Autodesk Inventor part; units mm, degrees
ref_plane "YZ Plane" through (0, 0, 0) normal (1, 0, 0) x (0, 1, 0)
ref_plane "XZ Plane" through (0, 0, 0) normal (0, 1, 0) x (-1, 0, 0)
ref_plane "XY Plane" through (0, 0, 0) normal (0, 0, 1) x (1, 0, 0)
sketch "スケッチ1" plane through (0, 0, 0) normal (0, 0, 1) x (1, 0, 0)
  circle A0 centre (0, 0) radius 17.9
  dimension "d0" = 35.8
extrude "押し出し1" add sketch "スケッチ1" against normal blind 3.3
fillet "フィレット1" radius 3 1 edges at (-17.9, 0, 0)
sketch "スケッチ2" plane through (0, 0, -3.3) normal (0, 0, -1) x (-1, 0, 0)
  circle A0 centre (0, 0) radius 19.25
  dimension "d4" = 38.5
extrude "押し出し2" add sketch "スケッチ2" along normal blind 38
sketch "スケッチ3" plane through (0, 0, -41.3) normal (0, 0, -1) x (-1, 0, 0)
  circle A0 centre (0, 0) radius 17.9
  dimension "d7" = 35.8
extrude "押し出し3" add sketch "スケッチ3" along normal blind 15.7
sketch "スケッチ4" plane through (0, 0, -57) normal (0, 0, -1) x (-1, 0, 0)
  circle A0 centre (0, 0) radius 1.585
  dimension "d10" = 3.17
extrude "押し出し4" add sketch "スケッチ4" along normal blind 10.7
sketch "スケッチ5" plane through (0, 0, 0) normal (0, 0, 1) x (1, 0, 0)
  circle A0 centre (0, 0) radius 1.585
  circle A1 centre (0, 0) radius 16
  dimension "d13" = 32
extrude "押し出し5" add sketch "スケッチ5" along normal blind 34.9 contours A0 | A1
chamfer "面取り1" distance 1 angle 45 1 edges at (-16, 0, 34.9)
sketch "スケッチ6" plane through (0, 0, 34.9) normal (0, 0, 1) x (1, 0, 0)
  circle A0 centre (0, 0) radius 10
  dimension "d19" = 20
extrude "押し出し6" add sketch "スケッチ6" along normal blind 3
sketch "スケッチ7" plane through (0, 0, 37.9) normal (0, 0, 1) x (1, 0, 0)
  circle A0 centre (0, 0) radius 1.585
  circle A1 centre (0, 0) radius 3
  dimension "d22" = 6
extrude "押し出し7" add sketch "スケッチ7" along normal blind 16.3 contours A0 | A1
sketch "スケッチ8" plane through (0, 0, 54.2) normal (0, 0, 1) x (1, 0, 0)
  circle A0 centre (0, 0) radius 3
  line L0 (-1.6583, 2.5) -> (1.6583, 2.5)
  arc A1 (1.6583, 2.5) -> (-1.6583, 2.5) centre (0, 0) ccw
  dimension "d25" = 2.5
extrude "押し出し8" cut sketch "スケッチ8" against normal blind 12 contours L0 A0 picked at (-0.1169, 2.6598)
sketch "スケッチ9" plane through (0, 0, 34.9) normal (0, 0, 1) x (1, 0, 0)
  circle A0 centre (0, 13) radius 1.25
  circle A1 centre (-13, 0) radius 1.25
  circle A2 centre (0, -13) radius 1.25
  circle A3 centre (13, 0) radius 1.25
  circle A4 centre (0, 0) radius 13 construction
  dimension "d28" = 2.5
  dimension "d29" = 2.5
  dimension "d30" = 2.5
  dimension "d31" = 2.5
  dimension "d32" = 26
extrude "押し出し9" cut sketch "スケッチ9" against normal blind 12
properties part number "RS-555-71"
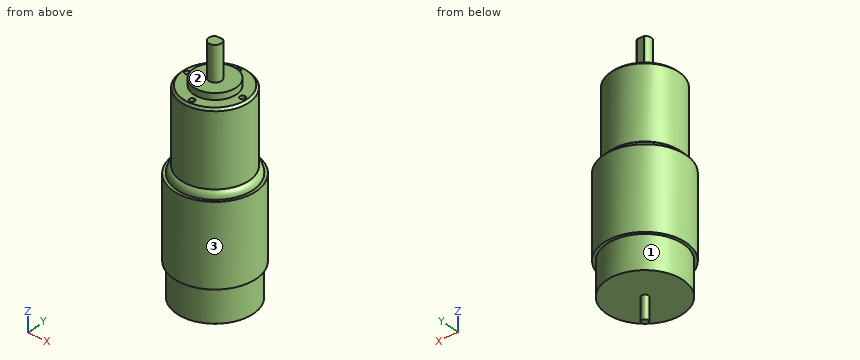
Model file for the job. Use its own axes, mm. Face numbers are marked on the shaded views. A direction names the side the tool comes from. Give positions to 0.01 mm unless a question says otherwise; leave off trailing zeros. Loops run counter-clockwise (first coordinate to the right, second up) from the corner with the lowest first, then second, coordinate; pieces in that order, holes last. Notation, with made-up numbers: (47.5, 76) - (87.5, 76) arc R27 cw to (87.5, 107) - close; hole circle Ø9 at (55, -33). An arc over 180 degrees is marked (long way). One line per item, written item: value. Start each with the question number.
1. Which spindle directions (+Z, -Z, +X, -X, +Y, -Y) get a long thin tool onto all of the face, cutting with end or side? Do the marked faces 1, 2 and 3. Say none if no direction does.
2. Pin check, flat tips, straight feed: pin 1 (2 mm diameter, centred on x = 13, y = 0, fed in from +Z); pin 2 (8 mm diameter, centred on x = 12, y = -6, fed in from +Z); pin 3 (1 mm diameter, centred on y = 5, z = 30.5, fed in from +X). Stop position of each tip, or through.
3. Slice it at B-B (z = -59). List the corners of the cut face in (x, y) (3 decimals), plus the area to 3 significant figures.
4. Slice it at A-A (z = -18.5). List the corners of the cut face in (x, y), plus the area to 3 significant figures.
5. Probe L1, parallel to Y at x = 0, z = 27; L2, parallel to X at y = -0.5, z = 24; L3, parallel to Z at x = -2.5, y = -3. List the from-to ranges inside material, lowest first. Write a range as from..to.
Solution:
1. face 1: -Z
1. face 2: +Z
1. face 3: +Z, -Z
2. pin 1: stops at z = 22.9
2. pin 2: stops at z = 37.9
2. pin 3: stops at x = 15.35
3. outline: circle Ø3.17 at (0, 0)
3. area: 7.89 mm^2
4. outline: circle Ø38.5 at (0, 0)
4. area: 1,160 mm^2
5. L1: y = -16..-14.25, -11.75..11.75, 14.25..16
5. L2: x = -15.99..-14.15, -11.85..11.85, 14.15..15.99
5. L3: z = -57..37.9
